Source: CAD feature listing. Evaluate the final solid. Frame: model axes, mm. A direction names the side the tool comes from. Give positions to 0.01 mm unless a question says otherwise; leave off trailing zeros. Order: outer loops, then holes, each group sorted by start corner. A loop starts at its lowest first (then second) coordinate and runs counter-clockwise, first axis right, second up. Notation, with made-up numbers: M -38,63.5 L 20,63.5 A18 ccw 20,85.5 Z; hole C 67.5,80 d6. An arc over 180 degrees is marked long. Answer in a Markdown table with one row per item. Add a question column.
(1) Section query A-A, the plane z = 12. Return loops of the section in (x, y).
(2) Pin query (flat end, axial travel): P1, Ø3, axis at x = 10, y = 0, coming from the +Z side; P2, Ø10, axis at y = -37.5, z = 22, coming from the -X side; P3, Ø4, axis at x = 30, z = 23.5, coming from the -Y side; P4, Ø2, axis at x = 61, y = -83, coming from the -Z side. Return the tip coordinate at first contact, or that it passes through.
(3) Section query C-C, the plane y = 40. Return loops of the section in (x, z).
(4) Material intervals for line 1 along Y through (x, z) = (70, 16.4); line 2 along X through (y, z) = (-20, 17.85); line 3 along Y through (x, z) = (50, 17), sorted ascending.
(5) Set-up query: faces 1 (the face through (75.312, -24, 7)), 2 (the face through (-20, 15, 17)), 3 (the face through (-23, -25, 0)). Return all of +Z, -Z, +X, -X, +Y, -Y with unobstructed straight access to the full face (end or side cutting, diameter ignored); none if empty.
(6) Mould query, pull axis X, two halves, no side actions, for faces 4 (the face through (27, 20, 17)), 5 (the face through (26, -50, 28)), 6 (the face through (45.417, -44.191, 26.479)), 7 (the face through (16.9, -33.17, 26.48)). Classes: pulls with the +X half, pulls with the -X half, needs draft (parallel to the pull), parting line crosses it, or undercut.
(7) Section query D-D, the plane y = 6.5. Return loops of the section in (x, z), plus the area to 3 significant figures.
(8) Section query B-B, the plane x = -10. Return loops of the section in (y, z).
Autodesk Fusion 360 part; units mm, degrees
sketch "Sketch1" plane through (0, 0, 0) normal (0, 0, 1) x (1, 0, 0)
  line L0 (-25, 50) -> (80, 50)
  line L1 (80, 50) -> (80, -100)
  line L2 (80, -100) -> (-25, -100)
  line L3 (-25, -100) -> (-25, 50)
  line L4 (-20, 45) -> (75, 45)
  line L5 (75, 45) -> (75, 25)
  line L6 (75, 25) -> (-20, 25)
  line L7 (-20, 25) -> (-20, 45)
  line L8 (-20, 20) -> (75, 20)
  line L9 (75, 20) -> (75, 10)
  line L10 (75, 10) -> (-20, 10)
  line L11 (-20, 10) -> (-20, 20)
  dimension "d1" = 105
  dimension "d2" = 150
extrude "Extrude1" add sketch "Sketch1" along normal blind 20 makes body 1
sketch "Sketch2" plane through (0, 0, 0) normal (0, 0, 1) x (1, 0, 0)
  line L0 (-20.26, 44.7118) -> (75.3115, 44.7118)
  line L1 (75.3115, 44.7118) -> (75.3115, -94.4537)
  line L2 (75.3115, -94.4537) -> (-20.26, -94.4537)
  line L3 (-20.26, -94.4537) -> (-20.26, 44.7118)
extrude "Extrude2" cut sketch "Sketch2" along normal blind 15 bodies 1
sketch "Sketch3" plane through (0, 0, 0) normal (0, 0, 1) x (1, 0, 0)
  circle A0 centre (70, 0) radius 2.5
  circle A1 centre (-10, 0) radius 2.5
  circle A2 centre (70, -90) radius 2.5
  circle A3 centre (-10, -90) radius 2.5
  circle A4 centre (50, 0) radius 2.5
  circle A5 centre (50, -20) radius 2.5
  circle A6 centre (70, -20) radius 2.5
  circle A7 centre (10, 0) radius 2.5
  circle A8 centre (-10, -20) radius 2.5
  circle A9 centre (10, -20) radius 2.5
  circle A10 centre (30, 0) radius 2.5
  circle A11 centre (30, -20) radius 2.5
  dimension "d7" = 5
  dimension "d8" = 5
  dimension "d9" = 5
  dimension "d10" = 5
  dimension "d11" = 5
  dimension "d12" = 5
  dimension "d13" = 5
  dimension "d14" = 5
  dimension "d15" = 5
  dimension "d16" = 5
  dimension "d17" = 5
  dimension "d18" = 5
extrude "Extrude3" cut sketch "Sketch3" along normal blind 40 bodies 1
thread "Thread1" thread offset 0 thread length 10
thread "Thread2" thread offset 0 thread length 10
thread "Thread3" thread offset 0 thread length 10
thread "Thread4" thread offset 0 thread length 10
thread "Thread5" thread offset 0 thread length 10
thread "Thread6" thread offset 0 thread length 10
thread "Thread7" thread offset 0 thread length 10
thread "Thread8" thread offset 0 thread length 10
thread "Thread9" thread offset 0 thread length 10
thread "Thread10" thread offset 0 thread length 10
thread "Thread11" thread offset 0 thread length 10
thread "Thread12" thread offset 0 thread length 10
sketch "Sketch4" plane through (0, 0, 0) normal (0, 0, 1) x (1, 0, 0)
  line L0 (-20, 10) -> (75.1056, 10)
  line L1 (75.1056, 10) -> (75.1056, -96.3646)
  line L2 (75.1056, -96.3646) -> (-20, -96.3646)
  line L3 (-20, -96.3646) -> (-20, 10)
extrude "Extrude1'" add sketch "Sketch4" along normal blind 10 separate body makes body 2 in component "Component"
move_body "Move1" bodies 2 to x (1, 0, 0) y (0, 1, 0) z (0, 0, 1) at (0, 0, 20) in component "Component"
extrude "Extrude2'" cut 1 faces at (43.4037, -60.9097, 30) along direction (0, 0, -1) blind 5 on bodies 2 bodies 2 in component "Component"
combine "Combine1" operation add target body 1 tool bodies 2
sketch "Sketch5" plane through (0, 0, 25) normal (0, 0, 1) x (-1, 0, 0)
  line L0 (20, 96.3646) -> (-75.1056, 96.3646)
  line L1 (-75.1056, 96.3646) -> (-75.1056, -10)
  line L2 (-75.1056, -10) -> (20, -10)
  line L3 (20, -10) -> (20, 96.3646)
  circle A0 centre (-20, 40) radius 7.5
  line L4 (-12.5, 40) -> (-12.5, 70)
  arc A1 (-12.5, 70) -> (-27.5528, 70) centre (-20.0264, 70) ccw
  line L5 (-27.5528, 70) -> (-27.5528, 36.787)
  line L6 (-27.5528, 36.787) -> (-25.1136, 34.5135)
  line L7 (-27.5528, 35.6503) -> (-34.6305, 35.6503)
  arc A2 (-39.1972, 56.8295) -> (-34.6305, 35.6503) centre (-34.6305, 46.7322) ccw
  arc A3 (-27.5528, 56.8295) -> (-39.1972, 56.8295) centre (-33.375, 43.9561) ccw
  line L8 (-27.5528, 36.787) -> (-27.5528, 56.8295)
  line L9 (-27.5528, 56.8295) -> (-27.5528, 35.6503)
  dimension "d49" = 15
extrude "Extrude4" add sketch "Sketch5" along normal blind 3 contours A0 | A0 L4 A1 L5 L6 L8 L9 | L5 L7 A2 A3 L8 L9 bodies 1
component "Component" placed x (1, 0, 0) y (0, 1, 0) z (0, 0, 1) at (0, 0, 0)
Values follow:
| question | item | result |
|---|---|---|
| 1 | outline | M -25,-100 L 80,-100 L 80,50 L -25,50 Z; hole M -20.26,-94.45 L 75.31,-94.45 L 75.31,44.71 L 75,44.71 L 75,45 L -20,45 L -20,44.71 L -20.26,44.71 Z |
| 2 | P1 | stops at z = 25 |
| 2 | P2 | stops at x = -25 |
| 2 | P3 | stops at y = -96.36 |
| 2 | P4 | stops at z = 15 |
| 3 | outline | M -25,0 L -20.26,0 L -20.26,15 L -20,15 L -20,20 L -25,20 Z; M 75,15 L 75.31,15 L 75.31,0 L 80,0 L 80,20 L 75,20 Z |
| 4 | line 1 | y = -100 to -92.5, -87.5 to -22.5, -17.5 to -2.5, 2.5 to 10, 20 to 25, 45 to 50 |
| 4 | line 2 | x = -25 to -12.5, -7.5 to 7.5, 12.5 to 27.5, 32.5 to 47.5, 52.5 to 67.5, 72.5 to 80 |
| 4 | line 3 | y = -100 to -22.5, -17.5 to -2.5, 2.5 to 10, 20 to 25, 45 to 50 |
| 5 | face 1 | -Z |
| 5 | face 2 | +Z, -Z |
| 5 | face 3 | -Z, +X, -X, +Y, -Y |
| 6 | face 4 | undercut |
| 6 | face 5 | needs draft |
| 6 | face 6 | pulls with the +X half |
| 6 | face 7 | parting line crosses it |
| 7 | outline | M -25,0 L -20.26,0 L -20.26,15 L 75.31,15 L 75.31,0 L 80,0 L 80,20 L 75.11,20 L 75.11,25 L -20,25 L -20,20 L -25,20 Z |
| 7 | area | 1,140 mm² |
| 8 | outline | M -100,0 L -94.45,0 L -94.45,15 L -92.5,15 L -92.5,20 L -87.5,20 L -87.5,15 L -22.5,15 L -22.5,20 L -17.5,20 L -17.5,15 L -2.5,15 L -2.5,20 L 2.5,20 L 2.5,15 L 10,15 L 10,25 L -96.36,25 L -96.36,20 L -100,20 Z; M 20,15 L 25,15 L 25,20 L 20,20 Z; M 45,0 L 50,0 L 50,20 L 45,20 Z |
